Verification items for the finished model (mm, model axes). Give positions to 0.01 mm unless a question says otherwise; leave off trailing zeros. Order: outer loops, then holes, each group sorted by start corner. A loop starts at its lowest first (then second) coordinate and runs counter-clockwise, first axis right, second up. Notation, with made-up numbers: (61, 3.25) -> (89, 3.25) arc R23 ccw to (89, 23.25) -> close; hole circle Ø6 at (20, 54). An arc over 180 degrees is marked (long way). One line per question, with ' | ' between items. Start each with the question number.
Q1. Section check A-A on y = 2.7. Record the cut outline in (x, z), plus the area to 3 significant figures.
Q2. Section check C-C on z = 0. Record the cut outline in (x, y).
Q3. Material ranges on probe 1 along Z at (x, y) = (0, 2.55); probe 2 along X at (y, z) = (1.6, 0); probe 3 along Z at (x, y) = (-2.75, 1.1), recorded low to high. Write a range as [from, to].
Q4. Section check D-D on z = -5.75. Record the cut outline in (x, y), plus the area to 3 significant figures.
Q5. Mould release check, pull along X, two halves, no side actions. Record for faces 1 (the flat face through (0, 0, -4)), 2 (the cylindrical face through (-2, 1.97, -6.22)), 3 (the cylindrical face through (2.579, 1.676, 1.978)): released by +X, released by -X, zero draft, split by the parting line, or undercut.
Q6. Section check B-B on x = 0. Record the cut outline in (y, z).
Autodesk Inventor part; units mm, degrees
ref_plane "YZ Plane" through (0, 0, 0) normal (1, 0, 0) x (0, 1, 0)
ref_plane "XZ Plane" through (0, 0, 0) normal (0, 1, 0) x (-1, 0, 0)
ref_plane "XY Plane" through (0, 0, 0) normal (0, 0, 1) x (1, 0, 0)
sketch "Sketch1" plane through (0, 0, 0) normal (0, 1, 0) x (-1, 0, 0)
  circle A0 centre (0, 0) radius 3.25
  circle A1 centre (0, 0) radius 5.25
  line L0 (1.5, -5.0312) -> (-1.5, -5.0312)
  line L1 (-1.5, -5.0312) -> (-1.5, -10.0312)
  line L2 (-1.5, -10.0312) -> (1.5, -10.0312)
  line L3 (1.5, -10.0312) -> (1.5, -5.0312)
  line L4 (0, 0) -> (0, -10.0312)
  arc A2 (3.6415, -3.7818) -> (1.5, -9.0312) centre (8.4969, -8.8241) ccw
  arc A3 (-1.5, -9.0312) -> (-3.6415, -3.7818) centre (-8.4969, -8.8241) ccw
  dimension "d0" = 6.5
  dimension "d1" = 2
  dimension "d2" = 1.5
  dimension "d3" = 5
  dimension "d4" = 7
  dimension "d5" = 4
  dimension "d6" = 7
extrude "Extrusion1" add sketch "Sketch1" along normal blind 4
sketch "Sketch2" plane through (0, 4, 0) normal (0, 1, 0) x (1, 0, 0)
  arc A0 (-3.6415, 3.7818) -> (-1.5, 9.0312) centre (-8.4969, 8.8241) ccw
  arc A1 (-3.6415, 3.7818) -> (3.6415, 3.7818) centre (0, 0) ccw
  arc A2 (1.5, 9.0312) -> (3.6415, 3.7818) centre (8.4969, 8.8241) ccw
  line L0 (1.5, 9.0312) -> (1.5, 10.0312)
  line L1 (1.5, 10.0312) -> (-1.5, 10.0312)
  line L2 (-1.5, 10.0312) -> (-1.5, 9.0312)
  circle A3 centre (0, 0) radius 3.25
  line L3 (-8.6908, -12.2142) -> (10.4061, -12.2142)
  line L4 (10.4061, -12.2142) -> (10.4061, 17.7463)
  line L5 (10.4061, 17.7463) -> (-8.6908, 17.7463)
  line L6 (-8.6908, 17.7463) -> (-8.6908, -12.2142)
fillet "Fillet2" radius 0.5 2 edges at (1.5, 2, -10.0312) (-1.5, 2, -10.0312)
chamfer "Chamfer1" distance 0.6 angle 45 1 edges at (3.25, 4, 0)
sketch "Sketch3" plane through (1.5, 0, -9.0312) normal (1, 0, 0) x (0, 0, -1)
  line L0 (-5.2494, 4) -> (0, 4) construction
  line L1 (-2, 6) -> (1, 6)
  line L2 (1, 0) -> (1, 4) construction
  line L3 (1, 6) -> (1, 4)
  line L4 (0, 4) -> (1, 4) construction
  line L5 (-6, 4) -> (-2, 6)
  line L6 (-6, 4) -> (1, 4)
  point P0 (-9.0312, 0)
  dimension "d9" = 2
  dimension "d10" = 7
  dimension "d11" = 3
equation "\"d6\" = d4"
properties part number "thumb_bolt_converter"
Filled in:
1) outline: (-3.64, -3.78) arc R7 cw to (-1.5, -9.03) -> (-1.5, -9.53) arc R0.5 ccw to (-1, -10.03) -> (1, -10.03) arc R0.5 ccw to (1.5, -9.53) -> (1.5, -9.03) arc R7 cw to (3.64, -3.78) arc R5.25 ccw (long way) to start; hole circle Ø6.5 at (0, 0) | area: 71.4 mm²
2) outline: (-5.25, 0) -> (-3.25, 0) -> (-3.25, 3.4) -> (-3.85, 4) -> (-5.25, 4) -> close; (3.25, 0) -> (5.25, 0) -> (5.25, 4) -> (3.85, 4) -> (3.25, 3.4) -> close
3) probe 1: [-10.03, -3.25], [3.25, 5.25] | probe 2: [-5.25, -3.25], [3.25, 5.25] | probe 3: [-4.83, -1.73], [1.73, 4.47]
4) outline: (-2.21, 0) -> (2.21, 0) -> (2.21, 4) -> (-2.21, 4) -> close | area: 17.7 mm²
5) face 1: zero draft | face 2: released by -X | face 3: undercut
6) outline: (0, -10.03) -> (4, -10.03) -> (4, -3.85) -> (3.4, -3.25) -> (0, -3.25) -> close; (0, 3.25) -> (3.4, 3.25) -> (4, 3.85) -> (4, 5.25) -> (0, 5.25) -> close
